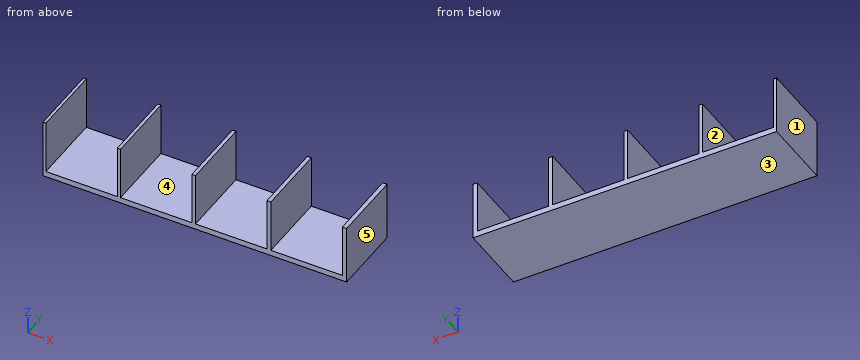
```python
from build123d import *

# Parameters (mm, degrees)
F0_W     = 85
F0_H     = 20
F1_DEPTH = 1.6
F2_W     = 0.8
F2_H     = 20
F2_W_2   = 0.9
F2_W_3   = 1
F2_W_4   = 1.1
F2_W_5   = 1.2
F3_DEPTH = 15


with BuildPart() as f1:
    # F0 (on Top) → F1 (new body)
    with BuildSketch(Plane.XY):
        with Locations((42.5, -10)):
            Rectangle(F0_W, F0_H)
    extrude(amount=F1_DEPTH)

    # F2 (on face) → F3 (join)
    with BuildSketch(Plane.XY.offset(1.6)):
        with Locations((0.4, -10)):
            Rectangle(F2_W, F2_H)
        with Locations((21.25, -10)):
            Rectangle(F2_W_2, F2_H)
        with Locations((42.2, -10)):
            Rectangle(F2_W_3, F2_H)
        with Locations((63.25, -10)):
            Rectangle(F2_W_4, F2_H)
        with Locations((84.4, -10)):
            Rectangle(F2_W_5, F2_H)
    extrude(amount=F3_DEPTH)


solid = f1.part
```
Source: CAD feature listing. Evaluate the final solid. Frame: model axes, mm. Face numbers are marked on the shaded views. A direction names the side the tool comes from. Give positions to 0.01 mm unless a question says otherwise; leave off trailing zeros. Write each loop counter-clockwise with the first axis right and the second up, starting at its lowest first coordinate (ties: lowest second). Pieces come first, ordered by that corner, then holes. Notation, with made-up numbers: (37, 78) - (85, 78) arc R20 ccw to (85, 92) - close; hole circle Ø2 at (70.5, 31). An arc over 180 degrees is marked (long way). One line per item, written item: value. Start each with the question number.
Q1. Section query C-C, the plane x = 65. Return the cut outline in (y, z).
Q2. Set-up query: the marked faces 4 and 5. Return all of +Z, -Z, +X, -X, +Y, -Y with unobstructed straight access to the full face (end or side cutting, diameter ignored); none if empty.
Q3. Section query B-B, the plane y = -8. Return the cut outline in (x, z), then the cut area to 3 significant figures.
Q4. Section query A-A, the plane z = 14.75. Return the cut outline in (x, y), then the cut area to 4 significant figures.
Q5. First-contact query: pin 1 Ø6 at (x, z) = (15.5, 6.5) entering from -Y; pin 2 Ø7.5 at (y, z) = (-12.5, 7.5) entering from -X; pin 3 Ø6 at (x, y) = (49, -13.5) entering from +Z. Flat tips, straight axial feed; report the tip coordinate or a pass-through.
Q6. Material intervals for probe 1 along X at (y, z) = (-8, 9); probe 2 along Z at (x, y) = (41, -17.5), sorted ascending. Write a range as from..to.
Q7. Draft query along X for the marked faces 1, 2 and 3. Return one class per face: +X half, -X half, draft (parallel to the pull), parting line (faces both ways), or undercut.
Answer:
1. outline: (-20, 0) - (0, 0) - (0, 1.6) - (-20, 1.6) - close
2. face 4: +Z, +Y, -Y
2. face 5: +Z, -Z, +X, +Y, -Y
3. outline: (0, 0) - (85, 0) - (85, 16.6) - (83.8, 16.6) - (83.8, 1.6) - (63.8, 1.6) - (63.8, 16.6) - (62.7, 16.6) - (62.7, 1.6) - (42.7, 1.6) - (42.7, 16.6) - (41.7, 16.6) - (41.7, 1.6) - (21.7, 1.6) - (21.7, 16.6) - (20.8, 16.6) - (20.8, 1.6) - (0.8, 1.6) - (0.8, 16.6) - (0, 16.6) - close
3. area: 211 mm2
4. outline: (0, -20) - (0.8, -20) - (0.8, 0) - (0, 0) - close; (20.8, -20) - (21.7, -20) - (21.7, 0) - (20.8, 0) - close; (41.7, -20) - (42.7, -20) - (42.7, 0) - (41.7, 0) - close; (62.7, -20) - (63.8, -20) - (63.8, 0) - (62.7, 0) - close; (83.8, -20) - (85, -20) - (85, 0) - (83.8, 0) - close
4. area: 100.0 mm2
5. pin 1: passes through
5. pin 2: stops at x = 0
5. pin 3: stops at z = 1.6
6. probe 1: x = 0..0.8, 20.8..21.7, 41.7..42.7, 62.7..63.8, 83.8..85
6. probe 2: z = 0..1.6
7. face 1: -X half
7. face 2: undercut
7. face 3: draft
